Here's how the part is built. I have some questions about the finished solid (model axes, mm). Face numbers are marked on the shaded views. A direction names the side the tool comes from. Round coordinates to 2 decimals unless told otherwise and drop trailing zeros. Order: outer loops, then holes, each group sorted by start corner. A loop starts at its lowest first (then second) coordinate and runs counter-clockwise, first axis right, second up. Notation, with made-up numbers: (80.5, 22.25) -> (100.5, 22.25) arc R18 cw to (100.5, 42.25) -> close; hole circle Ø4 at (52, -3). An arc over 180 degrees is marked (long way). Use a Markdown table: item, result. Add a question column.
(1) I want a section at D-D, the plane y = -9.25. Please give me the cut outline in (x, z) (3 decimals), then the cut area to 3 significant figures.
(2) If I drill on probe 1 along Y at (x, z) = (18.5, 0); probe 2 along Y at (x, z) = (16, 2); probe 3 along Z at (x, y) = (-19, -0.5), over which ranges is the centre line in solid material (lowest first)?
(3) On a 3-axis mill with a long thin cutter (end or side, diameter ignored), from which of +Z, -Z, +X, -X, +Y, -Y can I reach the whole of each face in a straight line? I mean the marked faces 4, 5, 6, 7 and 8. Say none if no direction works.
(4) I want a section at C-C, the plane x = 24. Please give me the cut outline in (y, z), then the cut area to 3 significant figures.
(5) Thinking about a two-plate mould opening in Z: for the marked faces 1, 2 and 3, which applies, pulls with the +Z half, pulls with the -Z half, needs draft (parallel to the pull), parting line crosses it, or undercut?
(6) I'm going to push flat-ended pins straight in: P1, Ø6, axis at x = 7.5, z = 18.5, coming from the +Y side; P2, Ø11.5, axis at x = 0, y = 0, coming from the -Z side; P3, Ø2, axis at x = -19.5, y = 3.5, coming from the +Z side. Where does each tip first touch, or does it pass through?
(7) I want a section at B-B, the plane z = -1. Please give me the cut outline in (x, y) (3 decimals).
from build123d import *

# Parameters (mm, degrees)
SKETCH1_R           = 12.7
SKETCH1_R_2         = 6.35
BOSS_EXTRUDE3_DEPTH = 27.305
SKETCH2_R           = 12.7
SKETCH2_R_2         = 6.35
BOSS_EXTRUDE4_DEPTH = 27.305


with BuildPart() as part:
    # Sketch1 → Boss-Extrude3 (new body, symmetric)
    with BuildSketch(Plane.XY):
        Circle(SKETCH1_R)
        Circle(SKETCH1_R_2, mode=Mode.SUBTRACT)
    extrude(amount=BOSS_EXTRUDE3_DEPTH, both=True)

    # Sketch2 → Boss-Extrude4 (add, symmetric)
    with BuildSketch(Plane(origin=(0, 0, 0), x_dir=(0, 0, -1), z_dir=(1, 0, 0))):
        Circle(SKETCH2_R)
        Circle(SKETCH2_R_2, mode=Mode.SUBTRACT)
    extrude(amount=BOSS_EXTRUDE4_DEPTH, both=True)


solid = part.part
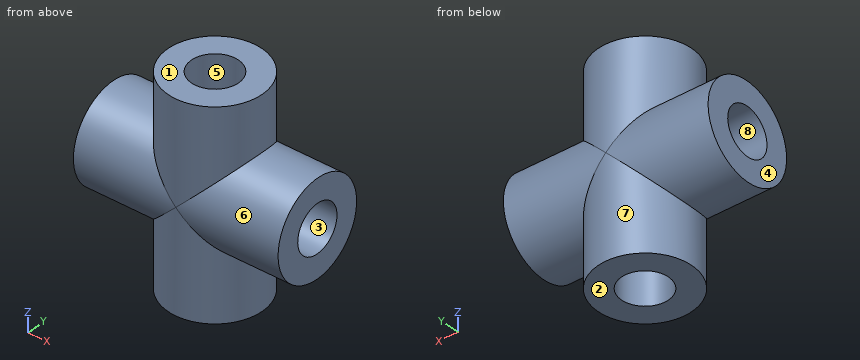
Taken from the geometry:
| question | item | result |
|---|---|---|
| 1 | outline | (-27.305, -8.702) -> (-8.702, -8.702) -> (-8.702, -27.305) -> (8.702, -27.305) -> (8.702, -8.702) -> (27.305, -8.702) -> (27.305, 8.702) -> (8.702, 8.702) -> (8.702, 27.305) -> (-8.702, 27.305) -> (-8.702, 8.702) -> (-27.305, 8.702) -> close |
| 1 | area | 1,600 mm2 |
| 2 | probe 1 | y = -12.7 to -6.35, 6.35 to 12.7 |
| 2 | probe 2 | y = -12.54 to -6.03, 6.03 to 12.54 |
| 2 | probe 3 | z = -12.69 to -6.33, 6.33 to 12.69 |
| 3 | face 4 | +Z, -Z, -X, +Y, -Y |
| 3 | face 5 | +Z |
| 3 | face 6 | +X |
| 3 | face 7 | -Z |
| 3 | face 8 | -X |
| 4 | outline | circle Ø25.4 at (0, 0); hole circle Ø12.7 at (0, 0) |
| 4 | area | 380 mm2 |
| 5 | face 1 | pulls with the +Z half |
| 5 | face 2 | pulls with the -Z half |
| 5 | face 3 | undercut |
| 6 | P1 | stops at y = 11.88 |
| 6 | P2 | stops at z = -12.7 |
| 6 | P3 | stops at z = 12.45 |
| 7 | outline | (-27.305, -12.661) -> (-1, -12.661) arc R12.7 ccw to (1, -12.661) -> (27.305, -12.661) -> (27.305, -6.271) -> (11.044, -6.271) arc R12.7 ccw to (11.044, 6.271) -> (27.305, 6.271) -> (27.305, 12.661) -> (1, 12.661) arc R12.7 ccw to (-1, 12.661) -> (-27.305, 12.661) -> (-27.305, 6.271) -> (-11.044, 6.271) arc R12.7 ccw to (-11.044, -6.271) -> (-27.305, -6.271) -> close; hole (-1, -6.271) -> (1, -6.271) arc R6.35 ccw to (1, 6.271) -> (-1, 6.271) arc R6.35 ccw to start |
